Autodesk Fusion 360 part; units mm, degrees
sketch "Sketch1" plane through (0, 0, 0) normal (0, 1, 0) x (1, 0, 0) in component "mountingPlatee"
  line L0 (0, 0) -> (110, 0)
  line L1 (110, 0) -> (110, -85)
  line L2 (110, -85) -> (0, -85)
  line L3 (0, -85) -> (0, 0)
  line L4 (15, -15) -> (95, -15)
  line L5 (95, -15) -> (95, -51)
  line L6 (95, -51) -> (15, -51)
  line L7 (15, -51) -> (15, -15)
  line L8 (15, -15) -> (15, -17.5)
  circle A0 centre (17.5, -17.5) radius 1.6
  line L9 (15, -51) -> (17.5, -51)
  line L10 (15, -48.5) -> (15, -51)
  circle A1 centre (17.5, -48.5) radius 1.6
  circle A2 centre (92.5, -48.5) radius 1.6
  circle A3 centre (92.5, -17.5) radius 1.6
  line L11 (15, -15) -> (20, -15)
  line L12 (20, -15) -> (20, -51)
  line L13 (20, -51) -> (15, -51)
  line L14 (15, -51) -> (15, -15)
  line L15 (95, -15) -> (88.7416, -15)
  line L16 (88.7416, -15) -> (88.7416, -51)
  line L17 (88.7416, -51) -> (95, -51)
  line L18 (95, -51) -> (95, -15)
  line L19 (22, -2.5) -> (88, -2.5)
  line L20 (88, -2.5) -> (88, -12.5)
  line L21 (88, -12.5) -> (22, -12.5)
  line L22 (22, -12.5) -> (22, -2.5)
  circle A4 centre (20, -70) radius 10
  circle A5 centre (5, -80) radius 1.6
  circle A6 centre (5, -5) radius 1.6
  circle A7 centre (105, -5) radius 1.6
  circle A8 centre (105, -80) radius 1.6
  line L23 (95, -68) -> (92, -68)
  line L24 (95, -75) -> (92, -75)
  line L25 (92, -71) -> (95, -71)
  line L26 (95, -72) -> (92, -72)
  line L27 (82, -68) -> (79, -68)
  line L28 (79, -71) -> (82, -71)
  line L29 (82, -71) -> (82, -68)
  line L30 (82, -72) -> (79, -72)
  line L31 (79, -75) -> (82, -75)
  line L32 (82, -75) -> (82, -72)
  line L33 (88, -2.5) -> (102, -2.5)
  line L34 (102, -2.5) -> (102, -12.5)
  line L35 (102, -12.5) -> (88, -12.5)
  line L36 (88, -12.5) -> (88, -2.5)
  circle A9 centre (20, -70) radius 11.1
  line L37 (92, -75) -> (96, -75)
  line L38 (96, -75) -> (96, -72)
  line L39 (96, -72) -> (92, -72)
  line L40 (92, -72) -> (92, -75)
  line L41 (92, -71) -> (96, -71)
  line L42 (96, -71) -> (96, -68)
  line L43 (96, -68) -> (92, -68)
  line L44 (92, -68) -> (92, -71)
  line L45 (82, -75) -> (78, -75)
  line L46 (78, -75) -> (78, -72)
  line L47 (78, -72) -> (82, -72)
  line L48 (82, -72) -> (82, -75)
  line L49 (82, -71) -> (78, -71)
  line L50 (78, -71) -> (78, -68)
  line L51 (78, -68) -> (82, -68)
  line L52 (82, -68) -> (82, -71)
  dimension "d3" = 110
  dimension "d4" = 85
  dimension "d5" = 80
  dimension "d6" = 36
  dimension "d9" = 3.2
  dimension "d12" = 3.2
  dimension "d15" = 3.2
  dimension "d16" = 3.2
  dimension "d24" = 3.2
  dimension "d25" = 3.2
  dimension "d26" = 3.2
  dimension "d27" = 3.2
  dimension "d30" = 14
  dimension "d31" = 10
  dimension "d32" = 22.2
sketch "Sketch1 (2)" plane through (0, 0, 0) normal (0, 1, 0) x (1, 0, 0)
sketch "Sketch2" plane through (0, 0, 0) normal (0, 1, 0) x (1, 0, 0)
extrude "Extrude1" add sketch "Sketch1" along normal blind 5 contours L0 L1 L2 L3 | L4 L6 L7 L8 L9 L10 L11 L12 L13 L14 | L4 L5 L6 L15 L16 L17 L18 | L19 L20 L21 L22 L36 | A9
sketch "Sketch3" plane through (0, 5, 0) normal (0, 1, 0) x (-1, 0, 0)
  line L0 (-92, 75) -> (-92, 72)
  line L1 (-92, 72) -> (-96, 72)
  line L2 (-96, 72) -> (-96, 75)
  line L3 (-96, 75) -> (-92, 75)
  circle A0 centre (-5, 5) radius 1.6
  circle A1 centre (-17.5, 17.5) radius 1.6
  line L4 (-102, 12.5) -> (-88, 12.5)
  line L5 (-88, 12.5) -> (-88, 2.5)
  line L6 (-88, 2.5) -> (-102, 2.5)
  line L7 (-102, 2.5) -> (-102, 12.5)
  circle A2 centre (-105, 5) radius 1.6
  circle A3 centre (-105, 80) radius 1.6
  circle A4 centre (-17.5, 48.5) radius 1.6
  line L8 (-92, 71) -> (-92, 68)
  line L9 (-92, 68) -> (-96, 68)
  line L10 (-96, 68) -> (-96, 71)
  line L11 (-96, 71) -> (-92, 71)
  circle A5 centre (-5, 80) radius 1.6
  line L12 (-78, 68) -> (-82, 68)
  line L13 (-82, 68) -> (-82, 71)
  line L14 (-82, 71) -> (-78, 71)
  line L15 (-78, 71) -> (-78, 68)
  circle A6 centre (-92.5, 17.5) radius 1.6
  line L16 (-78, 72) -> (-82, 72)
  line L17 (-82, 72) -> (-82, 75)
  line L18 (-82, 75) -> (-78, 75)
  line L19 (-78, 75) -> (-78, 72)
  line L20 (-20, 51) -> (-20, 15)
  line L21 (-20, 15) -> (-88.7416, 15)
  line L22 (-88.7416, 15) -> (-88.7416, 51)
  line L23 (-88.7416, 51) -> (-20, 51)
  circle A7 centre (-92.5, 48.5) radius 1.6
  circle A8 centre (-20, 70) radius 10
  line L24 (0, 85) -> (-110, 85)
  line L25 (-110, 85) -> (-110, 0)
  line L26 (-110, 0) -> (0, 0)
  line L27 (0, 0) -> (0, 85)
  line L28 (-88, 2.5) -> (-22, 2.5)
  line L29 (-22, 2.5) -> (-22, 12.5)
  line L30 (-22, 12.5) -> (-88, 12.5)
  line L31 (-88, 12.5) -> (-88, 2.5)
  circle A9 centre (-20, 70) radius 11.1
  dimension "d35" = 66
  dimension "d36" = 22.2
extrude "Extrude2" cut sketch "Sketch3" against normal blind 2 contours L5 L28 L29 L30 L31 | A9
extrude "Extrude3" cut 1 faces at (30.692, 3, 70.5515) along direction (0, -1, 0) blind 1
sketch "Sketch4" plane through (0, 5, 0) normal (0, 1, 0) x (-1, 0, 0)
  line L0 (-22, 2.5) -> (-102, 2.5)
  line L1 (-102, 2.5) -> (-102, 12.5)
  line L2 (-102, 12.5) -> (-22, 12.5)
  line L3 (-22, 12.5) -> (-22, 2.5)
  circle A0 centre (-20, 70) radius 11.1
  line L4 (-92, 75) -> (-92, 72)
  line L5 (-92, 72) -> (-96, 72)
  line L6 (-96, 72) -> (-96, 75)
  line L7 (-96, 75) -> (-92, 75)
  circle A1 centre (-5, 5) radius 1.6
  circle A2 centre (-17.5, 17.5) radius 1.6
  circle A3 centre (-105, 5) radius 1.6
  circle A4 centre (-105, 80) radius 1.6
  circle A5 centre (-17.5, 48.5) radius 1.6
  line L8 (-92, 71) -> (-92, 68)
  line L9 (-92, 68) -> (-96, 68)
  line L10 (-96, 68) -> (-96, 71)
  line L11 (-96, 71) -> (-92, 71)
  circle A6 centre (-5, 80) radius 1.6
  line L12 (-78, 68) -> (-82, 68)
  line L13 (-82, 68) -> (-82, 71)
  line L14 (-82, 71) -> (-78, 71)
  line L15 (-78, 71) -> (-78, 68)
  circle A7 centre (-92.5, 17.5) radius 1.6
  line L16 (-78, 72) -> (-82, 72)
  line L17 (-82, 72) -> (-82, 75)
  line L18 (-82, 75) -> (-78, 75)
  line L19 (-78, 75) -> (-78, 72)
  line L20 (-20, 51) -> (-20, 15)
  line L21 (-20, 15) -> (-88.7416, 15)
  line L22 (-88.7416, 15) -> (-88.7416, 51)
  line L23 (-88.7416, 51) -> (-20, 51)
  circle A8 centre (-92.5, 48.5) radius 1.6
  line L24 (0, 85) -> (-110, 85)
  line L25 (-110, 85) -> (-110, 0)
  line L26 (-110, 0) -> (0, 0)
  line L27 (0, 0) -> (0, 85)
  line L28 (-20, 15) -> (-15, 15)
  line L29 (-15, 15) -> (-15, 51)
  line L30 (-15, 51) -> (-20, 51)
  line L31 (-20, 51) -> (-20, 15)
  line L32 (-88.7416, 15) -> (-96, 15)
  line L33 (-96, 15) -> (-96, 51)
  line L34 (-96, 51) -> (-88.7416, 51)
  line L35 (-88.7416, 51) -> (-88.7416, 15)
  line L36 (-88.7416, 51) -> (-88.7416, 40)
  line L37 (-88.7416, 40) -> (-96, 40)
  line L38 (-96, 40) -> (-96, 26)
  line L39 (-96, 26) -> (-88.7416, 26)
  line L40 (-88.7416, 26) -> (-88.7416, 40)
extrude "Extrude4" cut sketch "Sketch4" against normal blind 5 contours L22 L33 L35 L37 L38 L39 L40
sketch "Sketch5" plane through (0, 5, 0) normal (0, 1, 0) x (-1, 0, 0)
  line L0 (-96, 40) -> (-88.7416, 40)
  line L1 (-88.7416, 40) -> (-88.7416, 51)
  line L2 (-88.7416, 51) -> (-20, 51)
  line L3 (-20, 51) -> (-20, 15)
  line L4 (-20, 15) -> (-88.7416, 15)
  line L5 (-88.7416, 15) -> (-88.7416, 26)
  line L6 (-88.7416, 26) -> (-96, 26)
  line L7 (-96, 26) -> (-96, 40)
  line L8 (-22, 2.5) -> (-102, 2.5)
  line L9 (-102, 2.5) -> (-102, 12.5)
  line L10 (-102, 12.5) -> (-22, 12.5)
  line L11 (-22, 12.5) -> (-22, 2.5)
  circle A0 centre (-20, 70) radius 11.1
  line L12 (-92, 75) -> (-92, 72)
  line L13 (-92, 72) -> (-96, 72)
  line L14 (-96, 72) -> (-96, 75)
  line L15 (-96, 75) -> (-92, 75)
  circle A1 centre (-5, 5) radius 1.6
  circle A2 centre (-17.5, 17.5) radius 1.6
  circle A3 centre (-105, 5) radius 1.6
  circle A4 centre (-105, 80) radius 1.6
  circle A5 centre (-17.5, 48.5) radius 1.6
  line L16 (-92, 71) -> (-92, 68)
  line L17 (-92, 68) -> (-96, 68)
  line L18 (-96, 68) -> (-96, 71)
  line L19 (-96, 71) -> (-92, 71)
  circle A6 centre (-5, 80) radius 1.6
  line L20 (-78, 68) -> (-82, 68)
  line L21 (-82, 68) -> (-82, 71)
  line L22 (-82, 71) -> (-78, 71)
  line L23 (-78, 71) -> (-78, 68)
  circle A7 centre (-92.5, 17.5) radius 1.6
  line L24 (-78, 72) -> (-82, 72)
  line L25 (-82, 72) -> (-82, 75)
  line L26 (-82, 75) -> (-78, 75)
  line L27 (-78, 75) -> (-78, 72)
  circle A8 centre (-92.5, 48.5) radius 1.6
  line L28 (0, 85) -> (-110, 85)
  line L29 (-110, 85) -> (-110, 0)
  line L30 (-110, 0) -> (0, 0)
  line L31 (0, 0) -> (0, 85)
  line L32 (-20, 15) -> (-14.5, 15)
  line L33 (-14.5, 15) -> (-14.5, 51)
  line L34 (-14.5, 51) -> (-20, 51)
  line L35 (-20, 51) -> (-20, 15)
  line L36 (-88.7416, 15) -> (-97, 15)
  line L37 (-97, 15) -> (-97, 26)
  line L38 (-97, 26) -> (-88.7416, 26)
  line L39 (-88.7416, 26) -> (-88.7416, 15)
  line L40 (-88.7416, 40) -> (-97, 40)
  line L41 (-97, 40) -> (-97, 51)
  line L42 (-97, 51) -> (-88.7416, 51)
  line L43 (-88.7416, 51) -> (-88.7416, 40)
  dimension "d43" = 5.5
  dimension "d44" = 36
extrude "Extrude5" cut sketch "Sketch5" against normal blind 2 contours L0 L1 L40 L41 L42 L43 | L5 L6 L36 L37 L38 L39 | L3 L32 L33 L34 L35
sketch "Sketch6" plane through (0, 5, 0) normal (0, 1, 0) x (-1, 0, 0)
  line L0 (-14.5, 15) -> (-97, 15)
  line L1 (-97, 15) -> (-97, 26)
  line L2 (-97, 26) -> (-96, 26)
  line L3 (-96, 26) -> (-96, 40)
  line L4 (-96, 40) -> (-97, 40)
  line L5 (-97, 40) -> (-97, 51)
  line L6 (-97, 51) -> (-20, 51)
  line L7 (-20, 51) -> (-14.5, 51)
  line L8 (-14.5, 51) -> (-14.5, 15)
  line L9 (-22, 2.5) -> (-102, 2.5)
  line L10 (-102, 2.5) -> (-102, 12.5)
  line L11 (-102, 12.5) -> (-22, 12.5)
  line L12 (-22, 12.5) -> (-22, 2.5)
  circle A0 centre (-20, 70) radius 11.1
  line L13 (-92, 75) -> (-92, 72)
  line L14 (-92, 72) -> (-96, 72)
  line L15 (-96, 72) -> (-96, 75)
  line L16 (-96, 75) -> (-92, 75)
  circle A1 centre (-5, 5) radius 1.6
  circle A2 centre (-105, 5) radius 1.6
  circle A3 centre (-105, 80) radius 1.6
  line L17 (-92, 71) -> (-92, 68)
  line L18 (-92, 68) -> (-96, 68)
  line L19 (-96, 68) -> (-96, 71)
  line L20 (-96, 71) -> (-92, 71)
  circle A4 centre (-5, 80) radius 1.6
  line L21 (-78, 68) -> (-82, 68)
  line L22 (-82, 68) -> (-82, 71)
  line L23 (-82, 71) -> (-78, 71)
  line L24 (-78, 71) -> (-78, 68)
  line L25 (-78, 72) -> (-82, 72)
  line L26 (-82, 72) -> (-82, 75)
  line L27 (-82, 75) -> (-78, 75)
  line L28 (-78, 75) -> (-78, 72)
  line L29 (0, 85) -> (-110, 85)
  line L30 (-110, 85) -> (-110, 0)
  line L31 (-110, 0) -> (0, 0)
  line L32 (0, 0) -> (0, 85)
  line L33 (-97, 26) -> (-96, 26)
  line L34 (-96, 26) -> (-96, 40)
  line L35 (-96, 40) -> (-97, 40)
  line L36 (-97, 40) -> (-97, 26)
extrude "Extrude6" cut sketch "Sketch6" against normal blind 5 contours L2 L3 L4 L33 L34 L35 L36
extrude "Extrude7" cut 1 faces at (42.9139, 1, 51) along direction (0, 0, 1) blind 0.3
extrude "Extrude8" cut 1 faces at (42.9139, 1, 15) along direction (0, 0, -1) blind 0.3
sketch "Sketch7" plane through (0, 5, 0) normal (0, 1, 0) x (-1, 0, 0)
  line L0 (-97, 14.7) -> (-97, 51.3)
  line L1 (-97, 51.3) -> (-20, 51.3)
  line L2 (-20, 51.3) -> (-14.5, 51.3)
  line L3 (-14.5, 51.3) -> (-14.5, 14.7)
  line L4 (-14.5, 14.7) -> (-97, 14.7)
  line L5 (0, 85) -> (-110, 85)
  line L6 (-110, 85) -> (-110, 0)
  line L7 (-110, 0) -> (0, 0)
  line L8 (0, 0) -> (0, 85)
  line L9 (-78, 72) -> (-82, 72)
  line L10 (-82, 72) -> (-82, 75)
  line L11 (-82, 75) -> (-78, 75)
  line L12 (-78, 75) -> (-78, 72)
  line L13 (-78, 68) -> (-82, 68)
  line L14 (-82, 68) -> (-82, 71)
  line L15 (-82, 71) -> (-78, 71)
  line L16 (-78, 71) -> (-78, 68)
  circle A0 centre (-5, 80) radius 1.6
  line L17 (-92, 71) -> (-92, 68)
  line L18 (-92, 68) -> (-96, 68)
  line L19 (-96, 68) -> (-96, 71)
  line L20 (-96, 71) -> (-92, 71)
  circle A1 centre (-105, 80) radius 1.6
  circle A2 centre (-105, 5) radius 1.6
  circle A3 centre (-5, 5) radius 1.6
  line L21 (-92, 75) -> (-92, 72)
  line L22 (-92, 72) -> (-96, 72)
  line L23 (-96, 72) -> (-96, 75)
  line L24 (-96, 75) -> (-92, 75)
  circle A4 centre (-20, 70) radius 11.1
  line L25 (-22, 2.5) -> (-102, 2.5)
  line L26 (-102, 2.5) -> (-102, 12.5)
  line L27 (-102, 12.5) -> (-22, 12.5)
  line L28 (-22, 12.5) -> (-22, 2.5)
component "mountingPlatee" placed x (1, 0, 0) y (0, 1, 0) z (0, 0, 1) at (0, 0, 0)
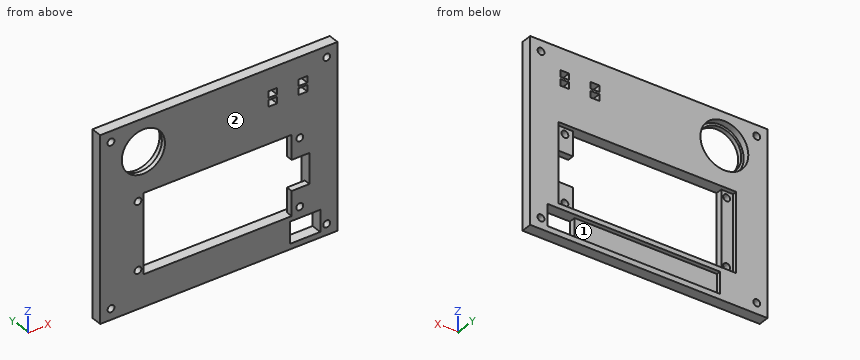
Model file for the job. Use its own axes, mm. Face numbers are marked on the shaded views. Give positions to 0.01 mm unless a question says otherwise; leave off trailing zeros. Order: outer loops, then holes, each group sorted by start corner. A loop starts at its lowest first (then second) coordinate and runs counter-clockwise, first axis right, second up. Notation, with made-up numbers: M 81,16 L 125,16 A23 cw 125,26 Z; hole C 24,-36.5 d4. An arc over 180 degrees is marked long. Write item = value, one per line.
Q1. Drill centre lines: line 1 (Z direction, x = 105, y = 3); line 2 (Z direction, x = 68, y = 3.8); line 3 (Z direction, x = 80, y = 0.3). Where is each one in solid material? Low to high. Write a range as [from, to].
Derived:
line_1 = [0, 3.4], [6.6, 78.4], [81.6, 85]
line_2 = [0, 2.5], [12.5, 14.7], [51.3, 85]
line_3 = [0, 14.7], [51.3, 68], [71, 72], [75, 85]
Q2. Cut at D-D, the plane x = 105. List the corners of the cut face in (y, z).
Derived:
outline = M 0,0 L 5,0 L 5,3.4 L 0,3.4 Z; M 0,6.6 L 5,6.6 L 5,78.4 L 0,78.4 Z; M 0,81.6 L 5,81.6 L 5,85 L 0,85 Z
Q3. Flat gauge pin, fed straight in: pin 1 (4 mm diameter, centred on x = 91.5, z = 46.5, fed in from +Y). Where does the tip first touch, or does it go through?
Derived:
pin_1 = 3
Q4. Cut at C-C, the plane y = 3.75. Count the separate pieces of the cut face and the enclosed holes in it, then the cut area to 3 significant figures.
Derived:
separate_pieces = 1
enclosed_holes = 11
area = 5,060 mm2
Q5. Cut at B-B, the plane z = 24.5. List the corners of the cut face in (x, y).
Derived:
outline = M 0,0 L 20,0 L 20,3 L 14.5,3 L 14.5,5 L 0,5 Z; M 88.74,0 L 110,0 L 110,5 L 97,5 L 97,3 L 88.74,3 Z
Q6. Cut at A-A, the plane x = 83.5. List the corners of the cut face in (y, z), then the cut area to 3 significant figures.
Derived:
outline = M 0,0 L 5,0 L 5,2.5 L 3,2.5 L 3,12.5 L 5,12.5 L 5,14.7 L 0,14.7 Z; M 0,51.3 L 5,51.3 L 5,85 L 0,85 Z
area = 222 mm2
Q7. Two-plate mould, pull along X, no slides. Class the marked faces 1 and 2: pulls with the +X half, pulls with the -X half, needs draft (parallel to the pull), parting line crosses it, or undercut.
Derived:
face_1 = undercut
face_2 = needs draft
